Autodesk Inventor part; units mm, degrees
ref_plane "YZ Plane" through (0, 0, 0) normal (1, 0, 0) x (0, 1, 0)
ref_plane "XZ Plane" through (0, 0, 0) normal (0, 1, 0) x (-1, 0, 0)
ref_plane "XY Plane" through (0, 0, 0) normal (0, 0, 1) x (1, 0, 0)
sketch "Sketch1" plane through (0, 0, 0) normal (0, 0, 1) x (1, 0, 0)
  circle A0 centre (0, 0) radius 1.5
  circle A1 centre (0, 0) radius 4.5
  line L0 (4.5, 0) -> (4.5, 4.5)
  line L1 (4.5, 4.5) -> (0, 4.5)
  line L2 (4.5, 0) -> (4.5, -4.5)
  line L3 (4.5, -4.5) -> (0, -4.5)
  dimension "d0" = 3
  dimension "d1" = 9
extrude "Extrusion1" add sketch "Sketch1" along normal blind 3
sketch "Sketch2" plane through (4.5, -4.5, 0) normal (1, 0, 0) x (0, 0, -1)
  line L0 (0, 0) -> (0, 9)
  line L1 (0, 9) -> (-3, 9)
  line L2 (-3, 0) -> (-3, 9)
  line L3 (0, 0) -> (-3, 0)
  line L4 (-3, 9) -> (-3, 0)
  line L5 (-3, 0) -> (-3, 4.5)
  line L6 (-3, 4.5) -> (-3, 34.5)
  line L7 (-3, 34.5) -> (17, 34.5)
  line L8 (17, 34.5) -> (17, -15.5)
  line L9 (17, -15.5) -> (-3, -15.5)
  line L10 (-3, -15.5) -> (-3, 4.5)
  point P0 (0, 4.5)
  dimension "d4" = 4.5
  dimension "d5" = 30
  dimension "d6" = 20
  dimension "d7" = 50
extrude "Extrusion2" add sketch "Sketch2" along normal blind 3
sketch "Sketch3" plane through (7.5, -4.5, 0) normal (1, 0, 0) x (0, 0, -1)
  line L0 (-3, -15.5) -> (17, -15.5)
  line L1 (17, -15.5) -> (17, 34.5)
  line L2 (17, 34.5) -> (-3, 34.5)
  line L3 (-3, 34.5) -> (-3, -15.5)
  line L4 (-3, 0) -> (-3, -15.5)
  line L5 (-3, -15.5) -> (0, -15.5)
  line L6 (-3, -15.5) -> (17, -15.5)
  line L7 (0, -15.5) -> (0, 34.5)
  line L8 (17, -15.5) -> (14, -15.5)
  line L9 (14, -15.5) -> (14, 34.5)
  line L10 (17, 34.5) -> (-3, 34.5)
  line L11 (0, -15.5) -> (0, 9.5)
  line L12 (0, 9.5) -> (0, 11)
  line L13 (0, 11) -> (14, 11)
  line L14 (14, 11) -> (14, 8)
  line L15 (14, 8) -> (0, 8)
  line L16 (0, 8) -> (0, 9.5)
  line L17 (0, 9.5) -> (0, -4.5)
  line L18 (0, -4.5) -> (0, -6)
  line L19 (0, -6) -> (14, -6)
  line L20 (14, -6) -> (14, -3)
  line L21 (14, -3) -> (0, -3)
  line L22 (0, 9.5) -> (0, 23.5)
  line L23 (0, 23.5) -> (0, 25)
  line L24 (0, 25) -> (14, 25)
  line L25 (14, 25) -> (14, 22)
  line L26 (14, 22) -> (0, 22)
  line L27 (0, -15.5) -> (4, -15.5)
  line L28 (4, -15.5) -> (4, 34.5)
  line L29 (14, -15.5) -> (10, -15.5)
  line L30 (10, -15.5) -> (10, 34.5)
  point P0 (0, 4.5)
  point P1 (10, -6)
  point P2 (4, -6)
  point P3 (10, -3)
  point P4 (10, 8)
  point P5 (4, 8)
  point P6 (4, -3)
  point P7 (10, 11)
  point P8 (10, 22)
  point P9 (4, 22)
  point P10 (4, 11)
  point P11 (10, 25)
  point P12 (4, 25)
  dimension "d10" = 3
  dimension "d11" = 3
  dimension "d12" = 25
  dimension "d13" = 1.5
  dimension "d14" = 3
  dimension "d15" = 14
  dimension "d16" = 1.5
  dimension "d17" = 3
  dimension "d18" = 14
  dimension "d19" = 1.5
  dimension "d20" = 3
  dimension "d21" = 4
  dimension "d22" = 4
extrude "Extrusion3" cut sketch "Sketch3" against normal blind 3 contours L28 L19 L30 L0 | L28 L15 L30 L21 | L2 L30 L24 L28 | L28 L26 L30 L13
sketch "Sketch4" plane through (7.5, -4.5, 0) normal (1, 0, 0) x (0, 0, -1)
  line L0 (10, -6) -> (10, -15.5)
  line L1 (10, -15.5) -> (17, -15.5)
  line L2 (17, -15.5) -> (17, 34.5)
  line L3 (17, 34.5) -> (10, 34.5)
  line L4 (10, 34.5) -> (10, 25)
  line L5 (10, 25) -> (4, 25)
  line L6 (4, 25) -> (4, 34.5)
  line L7 (4, 34.5) -> (-3, 34.5)
  line L8 (-3, 34.5) -> (-3, -15.5)
  line L9 (-3, -15.5) -> (4, -15.5)
  line L10 (4, -15.5) -> (4, -6)
  line L11 (4, -6) -> (10, -6)
  line L12 (4, -3) -> (4, 8)
  line L13 (4, 8) -> (10, 8)
  line L14 (10, 8) -> (10, -3)
  line L15 (10, -3) -> (4, -3)
  line L16 (4, 11) -> (4, 22)
  line L17 (4, 22) -> (10, 22)
  line L18 (10, 22) -> (10, 11)
  line L19 (10, 11) -> (4, 11)
  line L20 (-3, -15.5) -> (0.5, -15.5)
  line L21 (-3, -15.5) -> (4, -15.5)
  line L22 (0.5, -15.5) -> (0.5, -12)
  circle A0 centre (0.5, -12) radius 3.5
  line L23 (-3, -15.5) -> (-3, 9.5)
  line L24 (-3, 34.5) -> (-3, -15.5)
  line L25 (-3, 9.5) -> (5.4894, 9.5)
  circle A1 centre (0.5, 31) radius 3.5
  line L26 (-3, 9.5) -> (7, 9.5)
  line L27 (7, 9.5) -> (7, 17.879)
  circle A2 centre (13.5, -12) radius 3.5
  circle A3 centre (13.5, 31) radius 3.5
  point P0 (0, 4.5)
  point P1 (-3, 31)
  point P2 (0.5, 34.5)
  point P3 (4, 31)
  point P4 (10, 31)
  point P5 (13.5, 34.5)
  point P6 (17, 31)
  point P7 (17, -12)
  point P8 (13.5, -15.5)
  point P9 (10, -12)
  point P10 (-3, -12)
  point P11 (4, -12)
  dimension "d25" = 3.5
  dimension "d26" = 3.5
  dimension "d27" = 25
extrude "Extrusion4" cut sketch "Sketch4" against normal blind 3 contours A2 L1 L0 | L2 L1 A2 | L10 L9 A0 | A3 L3 L2 | L9 L8 A0 | A3 L4 L3 | L8 L7 A1 | L7 L6 A1
fillet "Fillet1" radius 2 1 edges at (4.5, 0, 0)
properties part number "agarre_izquierda"
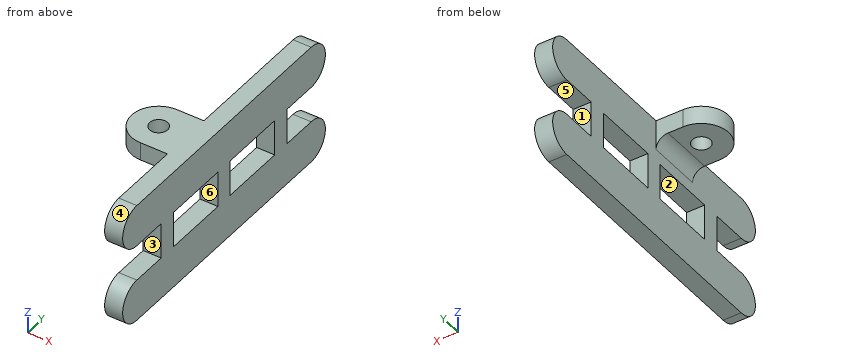
Build history of the part. All positions in model axes, mm. Face numbers are marked on the shaded views. A direction names the side the tool comes from. Coordinates: 2 decimals unless noted, no trailing zeros. Order: outer loops, then holes, each group sorted by start corner. A loop starts at its lowest first (then second) coordinate and runs counter-clockwise, first axis right, second up. Notation, with made-up numbers: (43.25, 7) - (64.25, 7) arc R7 ccw to (64.25, 12) - close; hole circle Ø11 at (23, 82.5). An arc over 180 degrees is marked (long way). Write each question's results on one line, items separated by ' | '. Start each with the question number.
Item 1: Band-saw the part on A-A on x = -0.75. Write the cut outline in (y, z).
Item 2: Band-saw the part on D-D on x = 5.75. Write the cut outline in (y, z), and give its area (3 significant figures).
Item 3: Tool access for the marked faces 1, 2 and 3: list every direction of +Z, -Z, +X, -X, +Y, -Y with a clear straight run to the whole face (end or side of a thin tool).
Item 4: Mould opens along Y. For the marked faces 4, 5 and 6 say: released by +Y, released by -Y, zero draft, split by the parting line, or undercut.
Item 5: Band-saw the part on C-C on z = -5.75. Write the cut outline in (x, y), and give its area (3 significant figures).
Item 6: Wall check: probe 1 along Z at (x, y) = (6.75, -4.5); probe 2 along Y at (x, z) = (0, 1.7); probe 3 along Y at (x, z) = (5, -5.5). Give the ranges that are in metal, low to high. Write a range as [from, to].
Item 7: Band-saw the part on B-B on y = -6.5. Write the cut outline in (x, z), and give its area (3 significant figures).
Item 8: Flat gauge pins, fed straight in: pin 1 (3.5 mm diameter, centred on x = 6.5, z = -6.5, fed in from -Y); pin 2 (5 mm diameter, centred on y = -3, z = -7, fed in from +X); pin 3 (5 mm diameter, centred on x = 1.5, z = 0, fed in from -Y); pin 4 (2 mm diameter, centred on x = -1.5, y = -1, fed in from -Z). Where does each tip first touch, or does it go through?
Numbers:
1) outline: (-4.44, 0) - (-1.3, 0) - (-1.3, 3) - (-4.44, 3) - close; (1.3, 0) - (4.44, 0) - (4.44, 3) - (1.3, 3) - close
2) outline: (-16.5, -17) - (26.5, -17) arc R3.5 ccw to (26.5, -10) - (20.5, -10) - (20.5, -4) - (26.5, -4) arc R3.5 ccw to (26.5, 3) - (-16.5, 3) arc R3.5 ccw to (-16.5, -4) - (-10.5, -4) - (-10.5, -10) - (-16.5, -10) arc R3.5 ccw to start; hole (-7.5, -10) - (3.5, -10) - (3.5, -4) - (-7.5, -4) - close; hole (6.5, -10) - (17.5, -10) - (17.5, -4) - (6.5, -4) - close | area: 733 mm^2
3) face 1: +X, -X, +Y | face 2: +X, -X | face 3: +X, -X, -Y
4) face 4: released by -Y | face 5: zero draft | face 6: undercut
5) outline: (4.5, -10.5) - (7.5, -10.5) - (7.5, -7.5) - (4.5, -7.5) - close; (4.5, 3.5) - (7.5, 3.5) - (7.5, 6.5) - (4.5, 6.5) - close; (4.5, 17.5) - (7.5, 17.5) - (7.5, 20.5) - (4.5, 20.5) - close | area: 27.0 mm^2
6) probe 1: [-17, -10], [-4, 3] | probe 2: [-4.5, -1.5], [1.5, 4.5] | probe 3: [-10.5, -7.5], [3.5, 6.5], [17.5, 20.5]
7) outline: (4.5, -17) - (7.5, -17) - (7.5, -10) - (4.5, -10) - close; (4.5, -4) - (7.5, -4) - (7.5, 3) - (4.5, 3) - close | area: 42.0 mm^2
8) pin 1: y = -10.5 | pin 2: through | pin 3: y = -4.5 | pin 4: z = 0
